Source: three-view drawing plus pictorial views. Frame: mm from the lowest corner of the part. Round coordinates to 2 decimals unless told otherwise and drop trailing zeros. Order: outer loops, then holes, each group sorted by start corner. A loop starts at its lowest first (then second) coordinate and runs counter-clockwise, first axis right, second up. Notation, with made-up numbers: M 63.25,-24 L 85.25,-24 A27 ccw 85.25,12 Z; hole C 74,80.25 d3. An arc over 180 degrees is marked long. Return JSON: item names as keys, results as strings. Group by question number.
Q1. Cut plane D-D on x = 5. Output: boundary loops of the cut face in (y, z), and give its area (3 significant figures).
Q2. Ray query, probe 1 along X at (y, z) = (0.6, 45); probe 2 along Z at (x, y) = (5, 0.45). Return the intervals inside material, ascending.
Q3. Cut plane C-C on z = 45. Output: boundary loops of the cut face in (x, y).
Q4. Cut plane B-B on y = 1.25. Output: boundary loops of the cut face in (x, z), and give its area (3 significant figures).
Q5. Cut plane A-A on x = 45. Output: boundary loops of the cut face in (y, z), and give its area (3 significant figures).
Q6. Contact query for flat-ended pins moving along their axis: pin 1 (0.6 mm diameter, centred on y = 1, z = 45, fed in from +X); pin 2 (1 mm diameter, centred on x = 49.5, y = 1.5, fed in from +Z); pin 3 (1 mm diameter, centred on y = 1.5, z = 42, fed in from -X). Output: stop coordinate, or through.
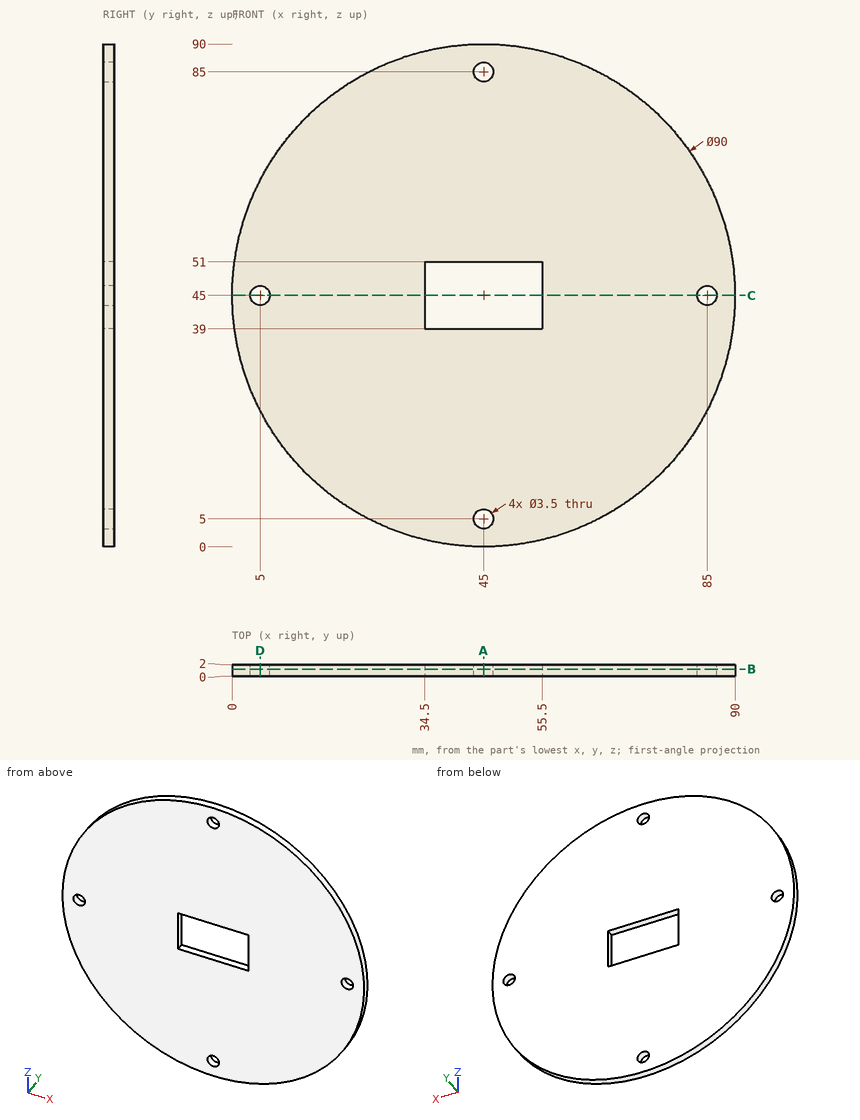
Result sheet:
{
 "1": {"outline": "M 0,24.38 L 2,24.38 L 2,43.25 L 0,43.25 Z; M 0,46.75 L 2,46.75 L 2,65.62 L 0,65.62 Z", "area": "75.5 mm²"},
 "2": {"probe 1": "x = 0 to 3.25, 6.75 to 34.5, 55.5 to 83.25, 86.75 to 90", "probe 2": "z = 24.38 to 43.25, 46.75 to 65.62"},
 "3": {"outline": "M 0,0 L 3.25,0 L 3.25,2 L 0,2 Z; M 6.75,0 L 34.5,0 L 34.5,2 L 6.75,2 Z; M 55.5,0 L 83.25,0 L 83.25,2 L 55.5,2 Z; M 86.75,0 L 90,0 L 90,2 L 86.75,2 Z"},
 "4": {"outline": "C 45,45 d90; hole C 5,45 d3.5; hole M 34.5,39 L 55.5,39 L 55.5,51 L 34.5,51 Z; hole C 45,5 d3.5; hole C 45,85 d3.5; hole C 85,45 d3.5", "area": "6,070 mm²"},
 "5": {"outline": "M 0,0 L 2,0 L 2,3.25 L 0,3.25 Z; M 0,6.75 L 2,6.75 L 2,39 L 0,39 Z; M 0,51 L 2,51 L 2,83.25 L 0,83.25 Z; M 0,86.75 L 2,86.75 L 2,90 L 0,90 Z", "area": "142 mm²"},
 "6": {"pin 1": "stops at x = 90", "pin 2": "stops at z = 89.82", "pin 3": "stops at x = 0.07"}
}
